Verification items for the finished model (mm, model axes). A direction names the side the tool comes from. Round coordinates to 2 decimals unless told otherwise and drop trailing zeros. Loops run counter-clockwise (first coordinate to the right, second up) from the corner with the lowest first, then second, coordinate; pieces in that order, holes last. Notation, with made-up numbers: (-36, -33.5) -> (9, -33.5) arc R21 cw to (9, 4.5) -> close; hole circle Ø5 at (22, 17.5). An arc over 180 degrees is marked (long way). Use a Markdown table: item, result. Add a question column.
Autodesk Inventor part; units mm, degrees
ref_plane "YZ Plane" through (0, 0, 0) normal (1, 0, 0) x (0, 1, 0)
ref_plane "XZ Plane" through (0, 0, 0) normal (0, 1, 0) x (-1, 0, 0)
ref_plane "XY Plane" through (0, 0, 0) normal (0, 0, 1) x (1, 0, 0)
sketch "Sketch1" plane through (0, 0, 0) normal (0, 0, 1) x (1, 0, 0)
  line L0 (-105, -80.9) -> (105, -80.9)
  line L1 (105, -80.9) -> (105, 80.9)
  line L2 (105, 80.9) -> (-105, 80.9)
  line L3 (-105, 80.9) -> (-105, -80.9)
  line L4 (-105, -80.9) -> (105, 80.9) construction
  line L5 (105, -80.9) -> (-105, 80.9) construction
  point P0 (0, 0)
  dimension "d0" = 210
  dimension "d1" = 161.8
extrude "Extrusion1" add sketch "Sketch1" along normal blind 5
sketch "Sketch3" plane through (0, 0, 0) normal (0, 0, -1) x (-1, 0, 0)
  line L0 (0.5, 69.9) -> (81.5, 69.9)
  line L1 (81.5, 69.9) -> (81.5, 20.9)
  line L2 (81.5, 20.9) -> (0.5, 20.9)
  line L3 (0.5, 20.9) -> (0.5, 69.9)
  line L4 (105, 80.9) -> (105, -80.9)
  line L5 (-105, 80.9) -> (105, 80.9)
  point P0 (0, 0)
  dimension "d20" = 49
  dimension "d21" = 81
  dimension "d22" = 23.5
  dimension "d23" = 11
hole "Hole2" at (-0.5, 69.9, 0) at (-81.5, 69.9, 0) at (-0.5, 20.9, 0) at (-81.5, 20.9, 0) direction (0, 0, 1) diameter 3 end through all countersink diameter 4 countersink angle 90
sketch "Sketch4" plane through (0, 0, 0) normal (0, 0, -1) x (-1, 0, 0)
  line L0 (-105, 80.9) -> (105, 80.9)
  circle A0 centre (81.5, 20.9) radius 2
  circle A1 centre (0.5, 20.9) radius 2
  circle A2 centre (81.5, 69.9) radius 2
  circle A3 centre (0.5, 69.9) radius 2
  line L1 (-105, -80.9) -> (-105, 80.9)
  line L2 (105, -80.9) -> (-105, -80.9)
  line L3 (105, 80.9) -> (105, -80.9)
  line L4 (-105, 80.9) -> (105, 80.9)
  line L5 (8.8, 80.9) -> (-8.8, 80.9)
  line L6 (-8.8, 80.9) -> (-8.8, 75.8)
  line L7 (-8.8, 75.8) -> (8.8, 75.8)
  line L8 (8.8, 75.8) -> (8.8, 80.9)
  line L9 (-26.2, 75.8) -> (-26.2, 80.9)
  line L10 (-26.2, 80.9) -> (-43.8, 80.9)
  line L11 (-43.8, 80.9) -> (-43.8, 75.8)
  line L12 (-43.8, 75.8) -> (-26.2, 75.8)
  line L13 (-61.2, 75.8) -> (-61.2, 80.9)
  line L14 (-61.2, 80.9) -> (-78.8, 80.9)
  line L15 (-78.8, 80.9) -> (-78.8, 75.8)
  line L16 (-78.8, 75.8) -> (-61.2, 75.8)
  line L17 (-96.2, 75.8) -> (-96.2, 80.9)
  line L18 (-96.2, 80.9) -> (-113.8, 80.9)
  line L19 (-113.8, 80.9) -> (-113.8, 75.8)
  line L20 (-113.8, 75.8) -> (-96.2, 75.8)
  line L21 (26.2, 80.9) -> (26.2, 75.8)
  line L22 (43.8, 80.9) -> (26.2, 80.9)
  line L23 (43.8, 75.8) -> (43.8, 80.9)
  line L24 (26.2, 75.8) -> (43.8, 75.8)
  line L25 (61.2, 80.9) -> (61.2, 75.8)
  line L26 (78.8, 80.9) -> (61.2, 80.9)
  line L27 (78.8, 75.8) -> (78.8, 80.9)
  line L28 (61.2, 75.8) -> (78.8, 75.8)
  line L29 (96.2, 80.9) -> (96.2, 75.8)
  line L30 (113.8, 80.9) -> (96.2, 80.9)
  line L31 (113.8, 75.8) -> (113.8, 80.9)
  line L32 (96.2, 75.8) -> (113.8, 75.8)
  line L33 (0, 0) -> (105, 0) construction
  point P0 (0, 75.8)
  point P1 (8.8, 80.9)
  point P2 (-8.8, 80.9)
  point P3 (0, 80.9)
  point P4 (-35, 80.9)
  point P5 (-35, 75.8)
  point P6 (-70, 80.9)
  point P7 (-70, 75.8)
  point P8 (-105, 80.9)
  point P9 (-105, 75.8)
  point P10 (35, 75.8)
  point P11 (35, 80.9)
  point P12 (70, 75.8)
  point P13 (70, 80.9)
  point P14 (105, 75.8)
  point P15 (105, 80.9)
  point P16 (-105, 75.8)
  point P17 (105, 75.8)
  dimension "d43" = 210
  dimension "d44" = 17.6
  dimension "d45" = 5.1
  dimension "d48" = 35
  dimension "d55" = 35
extrude "Extrusion2" cut sketch "Sketch4" against normal blind 10 contours L0 L17 L20 L1 | L0 L13 L16 L15 | L0 L9 L12 L11 | L32 L29 L0 L3 | L0 L8 L7 L6 | L27 L28 L25 L0 | L0 L23 L24 L21
sketch "Sketch5" plane through (0, 0, 0) normal (0, 0, -1) x (-1, 0, 0)
  line L0 (-105, -80.9) -> (-105, 80.9)
  line L1 (-105, 80.9) -> (26.2, 80.9)
  line L2 (-105, 48.49) -> (-99.9, 48.49)
  line L3 (-99.9, 48.49) -> (-99.9, 80.9)
  line L4 (-99.9, 80.9) -> (-105, 80.9)
  line L5 (-105, 80.9) -> (-105, 48.49)
  line L6 (-105, 16.23) -> (-99.9, 16.23)
  line L7 (-99.9, 16.23) -> (-99.9, -16.23)
  line L8 (-99.9, -16.23) -> (-105, -16.23)
  line L9 (-105, -16.23) -> (-105, 16.23)
  line L10 (-105, -80.9) -> (-99.9, -80.9)
  line L11 (-99.9, -80.9) -> (-99.9, -48.49)
  line L12 (-99.9, -48.49) -> (-105, -48.49)
  line L13 (-105, -48.49) -> (-105, -80.9)
  line L14 (-102.45, 48.49) -> (-102.45, 16.23) construction
  line L15 (-102.45, -48.49) -> (-102.45, -16.23) construction
  line L16 (0, 0) -> (0, 62.5) construction
  line L17 (105, -80.9) -> (105, 80.9)
  line L18 (105, 80.9) -> (96.35, 80.9)
  line L19 (105, 48.49) -> (99.9, 48.49)
  line L20 (99.9, 48.49) -> (99.9, 80.9)
  line L21 (99.9, 80.9) -> (105, 80.9)
  line L22 (105, 80.9) -> (105, 48.49)
  line L23 (105, 16.23) -> (99.9, 16.23)
  line L24 (99.9, 16.23) -> (99.9, -16.23)
  line L25 (99.9, -16.23) -> (105, -16.23)
  line L26 (105, -16.23) -> (105, 16.23)
  line L27 (105, -80.9) -> (99.9, -80.9)
  line L28 (99.9, -80.9) -> (99.9, -48.49)
  line L29 (99.9, -48.49) -> (105, -48.49)
  line L30 (105, -48.49) -> (105, -80.9)
  line L31 (102.45, 48.49) -> (102.45, 16.23) construction
  line L32 (102.45, -48.49) -> (102.45, -16.23) construction
  point P0 (-96.35, 80.9)
  point P1 (-99.9, 0)
  point P2 (-105, 0)
  point P3 (99.9, 0)
  point P4 (105, 0)
  point P5 (-105, -48.49)
  point P6 (-105, 16.23)
  point P7 (-105, -16.23)
  dimension "d37" = 32.46
  dimension "d38" = 161.8
  dimension "d39" = 5.1
  dimension "d40" = 32.26
extrude "Extrusion3" cut sketch "Sketch5" against normal blind 10
sketch "Sketch7" plane through (0, 0, 5) normal (0, 0, 1) x (1, 0, 0)
  line L0 (-105, -48.49) -> (105, -48.49)
  line L1 (8.8, -68.9) -> (-8.8, -68.9)
  line L2 (-8.8, -68.9) -> (-8.8, -80.9)
  line L3 (-8.8, -80.9) -> (8.8, -80.9)
  line L4 (8.8, -80.9) -> (8.8, -68.9)
  line L5 (-26.2, -80.9) -> (-26.2, -68.9)
  line L6 (-26.2, -68.9) -> (-43.8, -68.9)
  line L7 (-43.8, -68.9) -> (-43.8, -80.9)
  line L8 (-43.8, -80.9) -> (-26.2, -80.9)
  line L9 (-61.2, -80.9) -> (-61.2, -68.9)
  line L10 (-61.2, -68.9) -> (-78.8, -68.9)
  line L11 (-78.8, -68.9) -> (-78.8, -80.9)
  line L12 (-78.8, -80.9) -> (-61.2, -80.9)
  line L13 (-96.2, -80.9) -> (-96.2, -68.9)
  line L14 (-96.2, -68.9) -> (-113.8, -68.9)
  line L15 (-113.8, -68.9) -> (-113.8, -80.9)
  line L16 (-113.8, -80.9) -> (-96.2, -80.9)
  line L17 (26.2, -68.9) -> (26.2, -80.9)
  line L18 (43.8, -68.9) -> (26.2, -68.9)
  line L19 (43.8, -80.9) -> (43.8, -68.9)
  line L20 (26.2, -80.9) -> (43.8, -80.9)
  line L21 (61.2, -68.9) -> (61.2, -80.9)
  line L22 (78.8, -68.9) -> (61.2, -68.9)
  line L23 (78.8, -80.9) -> (78.8, -68.9)
  line L24 (61.2, -80.9) -> (78.8, -80.9)
  line L25 (96.2, -68.9) -> (96.2, -80.9)
  line L26 (113.8, -68.9) -> (96.2, -68.9)
  line L27 (113.8, -80.9) -> (113.8, -68.9)
  line L28 (96.2, -80.9) -> (113.8, -80.9)
  line L29 (-99.9, -80.9) -> (99.9, -80.9)
  point P0 (0, 0)
  point P1 (0, -80.9)
  point P2 (0, -48.49)
  point P3 (-35, -48.49)
  point P4 (-35, -80.9)
  point P5 (-70, -48.49)
  point P6 (-70, -80.9)
  point P7 (-105, -48.49)
  point P8 (-105, -80.9)
  point P9 (35, -80.9)
  point P10 (35, -48.49)
  point P11 (70, -80.9)
  point P12 (70, -48.49)
  point P13 (105, -80.9)
  point P14 (105, -48.49)
  point P15 (0, -80.9)
  point P16 (105, -48.49)
  dimension "d68" = 210
  dimension "d69" = 17.6
  dimension "d70" = 12
  dimension "d71" = 35
  dimension "d72" = 35
extrude "Extrusion4" cut sketch "Sketch7" against normal blind 10
sketch "Sketch8" plane through (0, 0, 5) normal (0, 0, 1) x (1, 0, 0)
  line L0 (-96.2, -68.9) -> (-96.2, -80.9)
  line L1 (-96.2, -75.9) -> (96.2, -75.9)
  line L2 (96.2, -80.9) -> (96.2, -68.9)
  line L3 (-96.2, -80.9) -> (-78.8, -80.9)
  line L4 (61.2, -80.9) -> (61.2, -68.9)
  line L5 (61.2, -68.9) -> (78.8, -68.9)
  line L6 (78.8, -68.9) -> (78.8, -80.9)
  line L7 (78.8, -80.9) -> (96.2, -80.9)
  line L8 (96.2, -80.9) -> (96.2, -68.9)
  line L9 (96.2, -68.9) -> (99.9, -68.9)
  line L10 (99.9, -68.9) -> (99.9, -48.49)
  line L11 (99.9, -48.49) -> (105, -48.49)
  line L12 (105, -48.49) -> (105, -16.23)
  line L13 (105, -16.23) -> (99.9, -16.23)
  line L14 (99.9, -16.23) -> (99.9, 16.23)
  line L15 (99.9, 16.23) -> (105, 16.23)
  line L16 (105, 16.23) -> (105, 48.49)
  line L17 (105, 48.49) -> (99.9, 48.49)
  line L18 (99.9, 48.49) -> (99.9, 75.8)
  line L19 (99.9, 75.8) -> (96.2, 75.8)
  line L20 (96.2, 75.8) -> (96.2, 80.9)
  line L21 (96.2, 80.9) -> (78.8, 80.9)
  line L22 (78.8, 80.9) -> (78.8, 75.8)
  line L23 (78.8, 75.8) -> (61.2, 75.8)
  line L24 (61.2, 75.8) -> (61.2, 80.9)
  line L25 (61.2, 80.9) -> (43.8, 80.9)
  line L26 (43.8, 80.9) -> (43.8, 75.8)
  line L27 (43.8, 75.8) -> (26.2, 75.8)
  line L28 (26.2, 75.8) -> (26.2, 80.9)
  line L29 (26.2, 80.9) -> (8.8, 80.9)
  line L30 (8.8, 80.9) -> (8.8, 75.8)
  line L31 (8.8, 75.8) -> (-8.8, 75.8)
  line L32 (-8.8, 75.8) -> (-8.8, 80.9)
  line L33 (-8.8, 80.9) -> (-26.2, 80.9)
  line L34 (-26.2, 80.9) -> (-26.2, 75.8)
  line L35 (-26.2, 75.8) -> (-43.8, 75.8)
  line L36 (-43.8, 75.8) -> (-43.8, 80.9)
  line L37 (-43.8, 80.9) -> (-61.2, 80.9)
  line L38 (-61.2, 80.9) -> (-61.2, 75.8)
  line L39 (-61.2, 75.8) -> (-78.8, 75.8)
  line L40 (-78.8, 75.8) -> (-78.8, 80.9)
  line L41 (-78.8, 80.9) -> (-96.2, 80.9)
  line L42 (-96.2, 80.9) -> (-96.2, 75.8)
  line L43 (-96.2, 75.8) -> (-99.9, 75.8)
  line L44 (-99.9, 75.8) -> (-99.9, 48.49)
  line L45 (-99.9, 48.49) -> (-105, 48.49)
  line L46 (-105, 48.49) -> (-105, 16.23)
  line L47 (-105, 16.23) -> (-99.9, 16.23)
  line L48 (-99.9, 16.23) -> (-99.9, -16.23)
  line L49 (-99.9, -16.23) -> (-105, -16.23)
  line L50 (-105, -16.23) -> (-105, -48.49)
  line L51 (-105, -48.49) -> (-99.9, -48.49)
  line L52 (-99.9, -48.49) -> (-99.9, -68.9)
  line L53 (-99.9, -68.9) -> (-96.2, -68.9)
  line L54 (-96.2, -68.9) -> (-96.2, -80.9)
  line L55 (-96.2, -80.9) -> (-78.8, -80.9)
  line L56 (-78.8, -80.9) -> (-78.8, -68.9)
  line L57 (-78.8, -68.9) -> (-61.2, -68.9)
  line L58 (-61.2, -68.9) -> (-61.2, -80.9)
  line L59 (-61.2, -80.9) -> (-43.8, -80.9)
  line L60 (-43.8, -80.9) -> (-43.8, -68.9)
  line L61 (-43.8, -68.9) -> (-26.2, -68.9)
  line L62 (-26.2, -68.9) -> (-26.2, -80.9)
  line L63 (-26.2, -80.9) -> (-8.8, -80.9)
  line L64 (-8.8, -80.9) -> (-8.8, -68.9)
  line L65 (-8.8, -68.9) -> (8.8, -68.9)
  line L66 (8.8, -68.9) -> (8.8, -80.9)
  line L67 (8.8, -80.9) -> (26.2, -80.9)
  line L68 (26.2, -80.9) -> (26.2, -68.9)
  line L69 (26.2, -68.9) -> (43.8, -68.9)
  line L70 (43.8, -68.9) -> (43.8, -80.9)
  line L71 (43.8, -80.9) -> (61.2, -80.9)
  point P0 (0, 0)
  point P1 (-78.8, -75.9)
  point P2 (78.8, -75.9)
  point P3 (-43.8, -75.9)
  point P4 (-61.2, -75.9)
  point P5 (-8.8, -75.9)
  point P6 (-26.2, -75.9)
  point P7 (61.2, -75.9)
  point P8 (43.8, -75.9)
  point P9 (26.2, -75.9)
  point P10 (8.8, -75.9)
  dimension "d77" = 5
extrude "Extrusion5" cut sketch "Sketch8" against normal blind 10 contours L1 L56 L3 L0 | L1 L60 L59 L58 | L1 L64 L63 L62 | L1 L68 L67 L66 | L68 L69 L70 L1 | L1 L4 L71 L70 | L1 L2 L7 L6
equation "\"d48\" = 0.166667 * d43"
equation "\"d55\" = 0.166667 * d43"
equation "\"d71\" = 0.166667 * d68"
equation "\"d72\" = 0.166667 * d68"
properties part number "FloorPlate_1" material "MDF Medium Density Fiberboard"
1) Go/stop test with flat-tipped pins: pin 1 (1.5 mm diameter, centred on y = -55, z = 2.5, fed in from +X); pin 2 (2.5 mm diameter, centred on x = -0.5, y = 20.9, fed in from +Z); pin 3 (2.5 mm diameter, centred on x = 67, z = 2.5, fed in from -Y); pin 4 (3 mm diameter, centred on y = -2.5, z = 2.5, fed in from -X). Record where each tip stops, or that it passes through.
2) Sectioned sample at A-A on z = 1.9. State how many separate pieces and enclosed holes the cut face has, then the cut area to 3 significant figures.
3) Sectioned sample at B-B on y = 63. Enter the section's corners in (x, z), then the cut area to 3 significant figures.
4) Release check for a two-part mould opening along Y. For faces 1 (the face through (88, 80.9, 2)), 2 (the face through (99.9, 0, 2)), 3 (the face through (-102, -48.49, 2)), 4 (the face through (-78.8, -72, 3)) record: released by +Y, released by -Y, zero draft, split by the parting line, or undercut.
5) Thickness scan on line 1 (X direction, y = 69.9, z = 3.3); line 2 (Y direction, x = -0.5, z = 3); line 3 (X direction, y = 20.9, z = 3.95). Record the ranges inside material, lowest first.
6) Access from +Z, -Z, +X, -X, +Y, -Y to the whole of each face (thin tool, end or side, straight path). Record for faces 5 (the face through (-96.2, -72, 3)), 6 (the face through (-78.8, 78, 2)), 7 (the face through (-96.2, 78, 2)).
Geometry results:
| question | item | result |
|---|---|---|
| 1 | pin 1 | x = 99.9 |
| 1 | pin 2 | through |
| 1 | pin 3 | y = -68.9 |
| 1 | pin 4 | x = -99.9 |
| 2 | separate pieces | 1 |
| 2 | enclosed holes | 4 |
| 2 | area | 30,800 mm^2 |
| 3 | outline | (-99.9, 0) -> (99.9, 0) -> (99.9, 5) -> (-99.9, 5) -> close |
| 3 | area | 999 mm^2 |
| 4 | face 1 | released by +Y |
| 4 | face 2 | undercut |
| 4 | face 3 | released by -Y |
| 4 | face 4 | zero draft |
| 5 | line 1 | -99.9 to -83, -80 to -2, 1 to 99.9 |
| 5 | line 2 | -68.9 to 19.4, 22.4 to 68.4, 71.4 to 75.8 |
| 5 | line 3 | -105 to -83, -80 to -2, 1 to 105 |
| 6 | face 5 | +Z, -Z, -X, -Y |
| 6 | face 6 | +Z, -Z, +Y |
| 6 | face 7 | +Z, -Z, -X, +Y |
